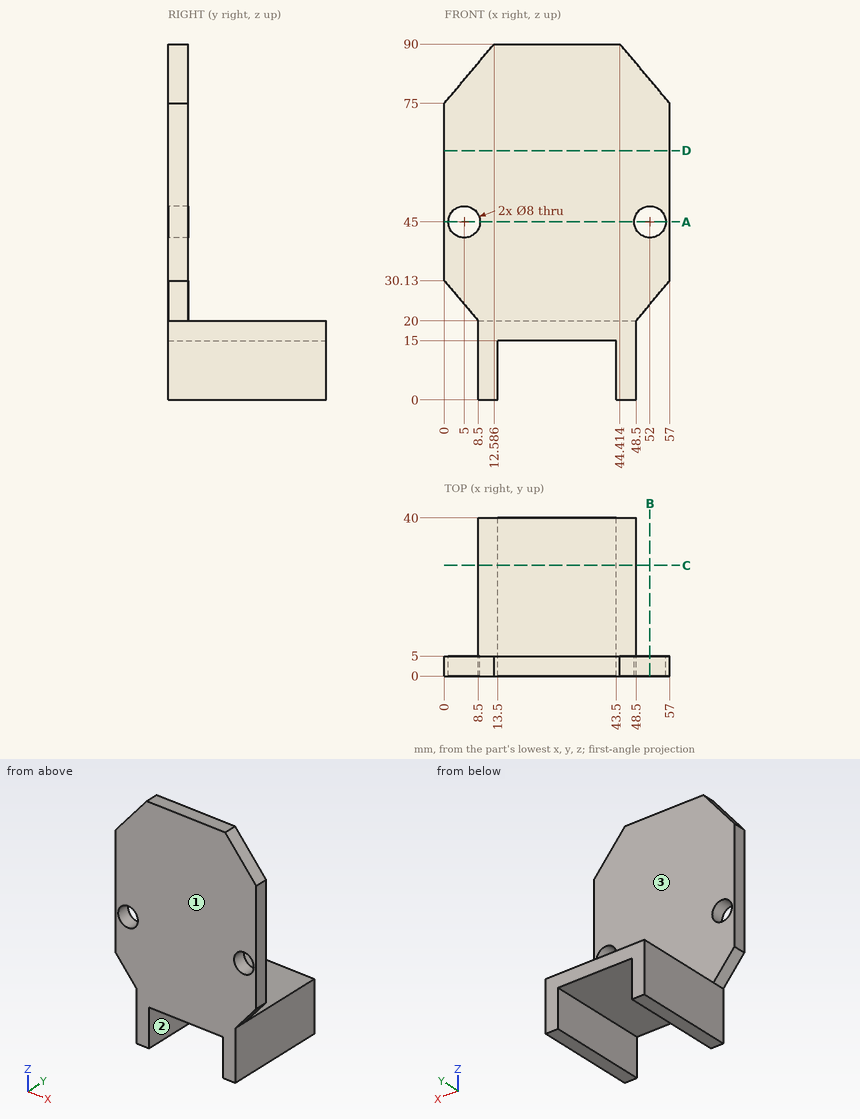
Study the drawing (mm; zero at the part's minimum x, y, z) and answer. A direction names the side the tool comes from. Coordinates: 2 decimals unless noted, no trailing zeros. Loops run counter-clockwise (first coordinate to the right, second up) from the corner with the lowest first, then second, coordinate; pieces in that order, holes last. Notation, with made-up numbers: (-37, 69.25) -> (-18, 69.25) arc R16 ccw to (-18, 90.25) -> close; hole circle Ø3 at (-36.75, -21). An arc over 180 degrees is marked (long way). Answer in a Markdown table with one row per item. Add a question column.
1. The part is cut by section D-D, the plane z = 63. Write down the section's boundary in (x, y).
2. The part is cut by section C-C, the plane y = 28. Write down the section's boundary in (x, z).
3. For the marked faces 1, 2 and 3, determine the directions among +Z, -Z, +X, -X, +Y, -Y from which every point of the face is accessible in a straight line to the end or side of a thin tool.
4. The part is cut by section B-B, the plane x = 52. Write down the section's boundary in (y, z).
5. Consider line 1 (X direction, y = 1.4, z = 45); line 2 (X direction, y = 11, z = 12); line 3 (Y direction, x = 25.5, z = 86.5). Determine where each line is inside the solid, lowest interval first. Write a range as [from, to].
6. Flat-ended cylindrical pins translate along their axes: P1, Ø17.5, axis at x = 23, y = 23, coming from the +Z side; P2, Ø6, axis at y = 28, z = 7.5, coming from the -X side; P3, Ø4.5, axis at y = 12, z = 6, coming from the +X side. Find the tip coordinate at first contact, or state that the pin passes through.
7. The part is cut by section A-A, the plane z = 45. Write down the section's boundary in (x, y).
Answer below:
| question | item | result |
|---|---|---|
| 1 | outline | (0, 0) -> (57, 0) -> (57, 5) -> (0, 5) -> close |
| 2 | outline | (8.5, 0) -> (13.5, 0) -> (13.5, 15) -> (43.5, 15) -> (43.5, 0) -> (48.5, 0) -> (48.5, 20) -> (8.5, 20) -> close |
| 3 | face 1 | +Z, -Z, +X, -X, -Y |
| 3 | face 2 | -Z, +Y, -Y |
| 3 | face 3 | +Z, +X, -X, +Y |
| 4 | outline | (0, 24.17) -> (5, 24.17) -> (5, 41) -> (0, 41) -> close; (0, 49) -> (5, 49) -> (5, 80.96) -> (0, 80.96) -> close |
| 5 | line 1 | [0, 1], [9, 48], [56, 57] |
| 5 | line 2 | [8.5, 13.5], [43.5, 48.5] |
| 5 | line 3 | [0, 5] |
| 6 | P1 | z = 20 |
| 6 | P2 | x = 8.5 |
| 6 | P3 | x = 48.5 |
| 7 | outline | (0, 0) -> (1, 0) -> (1, 5) -> (0, 5) -> close; (9, 0) -> (48, 0) -> (48, 5) -> (9, 5) -> close; (56, 0) -> (57, 0) -> (57, 5) -> (56, 5) -> close |
